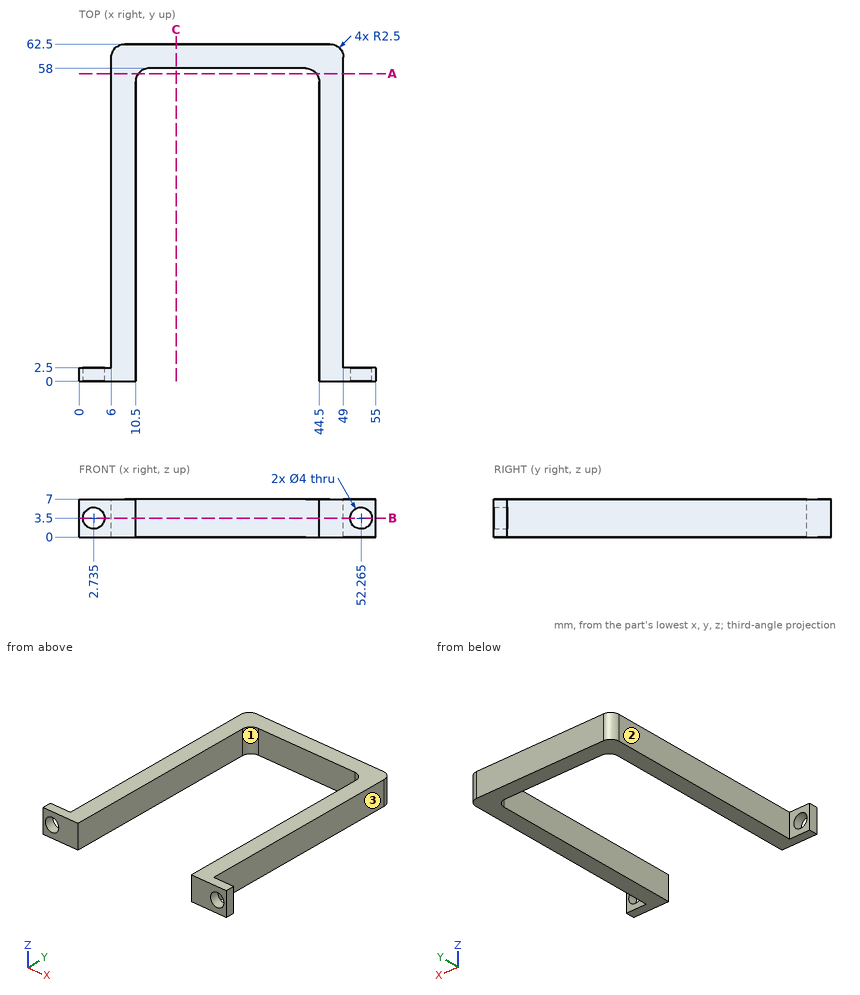
Check sheet for the drawn part. Datum: minimum x, y, z corner. Units: mm. A direction names the side the tool comes from. Round coordinates to 2 decimals unless told otherwise and drop trailing zeros. Loops run counter-clockwise (first coordinate to the right, second up) from the corner with the lowest first, then second, coordinate; pieces in that order, holes last. Notation, with made-up numbers: (85.25, -7.75) - (112.25, -7.75) arc R29 cw to (112.25, 26.25) - close; hole circle Ø10 at (60.25, 68). An arc over 180 degrees is marked (long way). Write item = value, one per line. Start each with the question number.
1. Thickness scan on line 1 (X direction, y = 15, z = 5.25); line 2 (Y direction, x = 26, z = 5.75); line 3 (X direction, y = 56, z = 4.5). Record the ranges inside material, lowest first.
2. Section check C-C on x = 18. Enter the section's corners in (y, z), then the cut area to 3 significant figures.
3. Section check A-A on y = 57. Enter the section's corners in (x, z).
4. Section check B-B on z = 3.5. Enter the section's corners in (x, y) (3 decimals).
5. Set-up check for the marked faces 1, 2 and 3: record each of +Z, -Z, +X, -X, +Y, -Y from which the full face is reachable in a straight line by a thin tool's end or side.
6. Depth check by flat-ended pin: pin 1 (3.5 mm diameter, centred on x = 28, z = 2.5, fed in from -Y); pin 2 (2 mm diameter, centred on y = 24, z = 3, fed in from +X); pin 3 (10 mm diameter, centred on x = 42, y = 7, fed in from +Z); pin 4 (3 mm diameter, centred on x = 52.265, z = 3.5, fed in from -Y). Enter the tip coordinate at first touch or a pass-through.
Working result:
q1.line_1 = 6 to 10.5, 44.5 to 49
q1.line_2 = 58 to 62.5
q1.line_3 = 6 to 10.55, 44.45 to 49
q2.outline = (58, 0) - (62.5, 0) - (62.5, 7) - (58, 7) - close
q2.area = 31.5 mm^2
q3.outline = (6, 0) - (11, 0) - (11, 7) - (6, 7) - close; (44, 0) - (49, 0) - (49, 7) - (44, 7) - close
q4.outline = (0, 0) - (0.735, 0) - (0.735, 2.5) - (0, 2.5) - close; (4.735, 0) - (10.5, 0) - (10.5, 55.5) arc R2.5 cw to (13, 58) - (42, 58) arc R2.5 cw to (44.5, 55.5) - (44.5, 0) - (50.265, 0) - (50.265, 2.5) - (49, 2.5) - (49, 60) arc R2.5 ccw to (46.5, 62.5) - (8.5, 62.5) arc R2.5 ccw to (6, 60) - (6, 2.5) - (4.735, 2.5) - close; (54.265, 0) - (55, 0) - (55, 2.5) - (54.265, 2.5) - close
q5.face_1 = +Z, -Z, -Y
q5.face_2 = +Z, -Z, -X, +Y
q5.face_3 = +Z, -Z, +X, +Y
q6.pin_1 = 58
q6.pin_2 = 49
q6.pin_3 = 7
q6.pin_4 = through
